The listing builds one solid part. Answer for the finished solid, in the listing's coordinates (mm). A direction names the side the tool comes from. Coordinates: 2 decimals unless noted, no trailing zeros. Order: outer loops, then holes, each group sorted by start corner. A loop starts at its lowest first (then second) coordinate and runs counter-clockwise, first axis right, second up. Notation, with made-up numbers: (45.5, 57.25) -> (54.5, 57.25) arc R25 cw to (54.5, 70.25) -> close; hole circle Ø5 at (72.5, 37). An arc over 180 degrees is marked (long way). Answer in a Markdown table with one row per item.
```python
from build123d import *

# Parameters (mm, degrees)
SKETCH_1_R          = 47
SKETCH_1_R_2        = 37
SKETCH_1_R_3        = 2.3
EXTRUDE_1_DEPTH     = 4
CUT_EXTRUDE_1_DEPTH = 5


with BuildPart() as part:
    # 草图1 → 凸台-拉伸1 (new body)
    with BuildSketch(Plane.XY):
        Circle(SKETCH_1_R)
        Circle(SKETCH_1_R_2, mode=Mode.SUBTRACT)
        with Locations((0, 42)):
            Circle(SKETCH_1_R_3, mode=Mode.SUBTRACT)
        with Locations((29.69848481, 29.69848481)):
            Circle(SKETCH_1_R_3, mode=Mode.SUBTRACT)
        with Locations((42, 0)):
            Circle(SKETCH_1_R_3, mode=Mode.SUBTRACT)
        with Locations((29.69848481, -29.69848481)):
            Circle(SKETCH_1_R_3, mode=Mode.SUBTRACT)
        with Locations((0, -42)):
            Circle(SKETCH_1_R_3, mode=Mode.SUBTRACT)
        with Locations((-29.69848481, -29.69848481)):
            Circle(SKETCH_1_R_3, mode=Mode.SUBTRACT)
        with Locations((-42, 0)):
            Circle(SKETCH_1_R_3, mode=Mode.SUBTRACT)
        with Locations((-29.69848481, 29.69848481)):
            Circle(SKETCH_1_R_3, mode=Mode.SUBTRACT)
    extrude(amount=EXTRUDE_1_DEPTH)

    # 草图3 → 切除-拉伸1 (cut, through all)
    with BuildSketch(Plane.XY.offset(4)):
        with BuildLine():
            ThreePointArc((23.893381773, 37.541394586), (17.02941274, 41.112639197), (9.65060241, 43.440946964))
            ThreePointArc((9.65060241, 43.440946964), (6.071396834, 41.162946208), (8.34939759, 37.583740632))
            ThreePointArc((8.34939759, 37.583740632), (14.733312146, 35.569362002), (20.671802208, 32.479633518))
            ThreePointArc((20.671802208, 32.479633518), (24.813472524, 33.399724269), (23.893381773, 37.541394586))
        make_face()
        with BuildLine():
            ThreePointArc((43.440946964, 9.65060241), (41.112639197, 17.02941274), (37.541394586, 23.893381773))
            ThreePointArc((37.541394586, 23.893381773), (33.399724269, 24.813472524), (32.479633518, 20.671802208))
            ThreePointArc((32.479633518, 20.671802208), (35.569362002, 14.733312146), (37.583740632, 8.34939759))
            ThreePointArc((37.583740632, 8.34939759), (41.162946208, 6.071396834), (43.440946964, 9.65060241))
        make_face()
        with BuildLine():
            ThreePointArc((37.541394586, -23.893381773), (41.112639197, -17.02941274), (43.440946964, -9.65060241))
            ThreePointArc((43.440946964, -9.65060241), (41.162946208, -6.071396834), (37.583740632, -8.34939759))
            ThreePointArc((37.583740632, -8.34939759), (35.569362002, -14.733312146), (32.479633518, -20.671802208))
            ThreePointArc((32.479633518, -20.671802208), (33.399724269, -24.813472524), (37.541394586, -23.893381773))
        make_face()
        with BuildLine():
            ThreePointArc((9.65060241, -43.440946964), (17.02941274, -41.112639197), (23.893381773, -37.541394586))
            ThreePointArc((23.893381773, -37.541394586), (24.813472524, -33.399724269), (20.671802208, -32.479633518))
            ThreePointArc((20.671802208, -32.479633518), (14.733312146, -35.569362002), (8.34939759, -37.583740632))
            ThreePointArc((8.34939759, -37.583740632), (6.071396834, -41.162946208), (9.65060241, -43.440946964))
        make_face()
        with BuildLine():
            ThreePointArc((-23.893381773, -37.541394586), (-17.02941274, -41.112639197), (-9.65060241, -43.440946964))
            ThreePointArc((-9.65060241, -43.440946964), (-6.071396834, -41.162946208), (-8.34939759, -37.583740632))
            ThreePointArc((-8.34939759, -37.583740632), (-14.733312146, -35.569362002), (-20.671802208, -32.479633518))
            ThreePointArc((-20.671802208, -32.479633518), (-24.813472524, -33.399724269), (-23.893381773, -37.541394586))
        make_face()
        with BuildLine():
            ThreePointArc((-43.440946964, -9.65060241), (-41.112639197, -17.02941274), (-37.541394586, -23.893381773))
            ThreePointArc((-37.541394586, -23.893381773), (-33.399724269, -24.813472524), (-32.479633518, -20.671802208))
            ThreePointArc((-32.479633518, -20.671802208), (-35.569362002, -14.733312146), (-37.583740632, -8.34939759))
            ThreePointArc((-37.583740632, -8.34939759), (-41.162946208, -6.071396834), (-43.440946964, -9.65060241))
        make_face()
        with BuildLine():
            ThreePointArc((-37.541394586, 23.893381773), (-41.112639197, 17.02941274), (-43.440946964, 9.65060241))
            ThreePointArc((-43.440946964, 9.65060241), (-41.162946208, 6.071396834), (-37.583740632, 8.34939759))
            ThreePointArc((-37.583740632, 8.34939759), (-35.569362002, 14.733312146), (-32.479633518, 20.671802208))
            ThreePointArc((-32.479633518, 20.671802208), (-33.399724269, 24.813472524), (-37.541394586, 23.893381773))
        make_face()
        with BuildLine():
            ThreePointArc((-9.65060241, 43.440946964), (-17.02941274, 41.112639197), (-23.893381773, 37.541394586))
            ThreePointArc((-23.893381773, 37.541394586), (-24.813472524, 33.399724269), (-20.671802208, 32.479633518))
            ThreePointArc((-20.671802208, 32.479633518), (-14.733312146, 35.569362002), (-8.34939759, 37.583740632))
            ThreePointArc((-8.34939759, 37.583740632), (-6.071396834, 41.162946208), (-9.65060241, 43.440946964))
        make_face()
    extrude(amount=-CUT_EXTRUDE_1_DEPTH, mode=Mode.SUBTRACT)


with BuildPart() as part_1:
    # Move Body 1: moved
    add(part.part.moved(Location((0, 0, -4))))


solid = part_1.part
```
(1) For a pull along Y with two mould halves and no side action, classify faces 1 (the flat face through (14, -35, 0)), 2 (the cylindrical face through (-41.154, -16.929, -1.972)) as released by +Y, released by -Y, zero draft, split by the parting line, or undercut.
Check values:
| item | result |
|---|---|
| face 1 | zero draft |
| face 2 | undercut |
(2) A cutting plane is placed at A-A, the plane y = 0. Determine the outline of the cut face in (x, z).
Check values:
| item | result |
|---|---|
| outline | (-47, -4) -> (-44.3, -4) -> (-44.3, 0) -> (-47, 0) -> close; (-39.7, -4) -> (-37, -4) -> (-37, 0) -> (-39.7, 0) -> close; (37, -4) -> (39.7, -4) -> (39.7, 0) -> (37, 0) -> close; (44.3, -4) -> (47, -4) -> (47, 0) -> (44.3, 0) -> close |
(3) Flat-ended cylindrical pins translate along their axes: pin 1 (1.5 mm diameter, centred on x = 19, z = -0.5, fed in from +Y); pin 2 (6 mm diameter, centred on x = 42, y = 0, fed in from -Z); pin 3 (1.5 mm diameter, centred on y = -8.5, z = -1.5, fed in from +X). Find the tip coordinate at first contact, or state that the pin passes through.
Check values:
| item | result |
|---|---|
| pin 1 | y = 43.31 |
| pin 2 | z = -4 |
| pin 3 | x = 46.36 |
(4) A cutting plane is placed at C-C, the plane z = -2.2. Count the separate pieces of the cut face and the enclosed holes in it, then the cut area to 3 significant figures.
Check values:
| item | result |
|---|---|
| separate pieces | 1 |
| enclosed holes | 17 |
| area | 1,590 mm² |
(5) Which of the six approach directions +Z, -Z, +X, -X, +Y, -Y give full straight-line access (tool end or side, diameter ignored) to faces 3 (the cylindrical face through (41.154, 16.929, -1.972)), 4 (the flat face through (14, -35, -4))?
Check values:
| item | result |
|---|---|
| face 3 | +Z, -Z |
| face 4 | -Z, +X, -X, +Y, -Y |
(6) Find the intervals of material crossed by line 1 along Y through (x, z) = (23, -3.5); line 2 along X through (y, z) = (-6.5, -1.1); line 3 along Y through (x, z) = (-14, -3.55), in increasing order. Write a range as from..to.
Check values:
| item | result |
|---|---|
| line 1 | -40.99..-38.1, -32.1..-28.98, 28.98..32.1, 38.1..40.99 |
| line 2 | -46.55..-42.17, -38.85..-36.42, 36.42..38.85, 42.17..46.55 |
| line 3 | -44.87..-42.24, -35.86..-34.25, 34.25..35.86, 42.24..44.87 |
